For this review, take the finished solid that the model builds, in its own axes (mm). Face numbers are marked on the shaded views. Round coordinates to 2 decimals unless told otherwise and drop trailing zeros. Order: outer loops, then holes, each group sorted by start corner. A loop starts at its lowest first (then second) coordinate and runs counter-clockwise, first axis right, second up.
from build123d import *

# Parameters (mm, degrees)
F0_W      = 45
F0_H      = 21
F0_R      = 2.25
F1_DEPTH  = 2
F2_DEPTH  = 37
F3_R      = 2.25
F4_DEPTH  = 2
F5_DEPTH  = 2
F6_R      = 3.4
F10_DEPTH = 25.29364
F11_R     = 3.4
F12_DEPTH = 13.84716
F13_DEPTH = 13.90348


with BuildPart() as f1:
    # F0 (on Top) → F1 (new body)
    with BuildSketch(Plane.XY):
        Rectangle(F0_W, F0_H)
        with Locations((-15, 0)):
            Circle(F0_R, mode=Mode.SUBTRACT)
        with Locations((15, 0)):
            Circle(F0_R, mode=Mode.SUBTRACT)
    extrude(amount=F1_DEPTH)

    # F0 (on Top) → F2 (join)
    with BuildSketch(Plane.XY):
        Polygon((22.5, 19.5), (22.5, 10.5), (22.5, -10.5), (24.5, -10.5), (24.5, 19.5), align=None)
    extrude(amount=F2_DEPTH)

    # F3 (on face) → F4 (cut)
    with BuildSketch(Plane(origin=(22.5, 0, 0), x_dir=(0, -1, 0), z_dir=(-1, 0, 0))):
        with Locations((0, 30.371862)):
            Circle(F3_R)
    extrude(amount=-F4_DEPTH, mode=Mode.SUBTRACT)

    # F3 (on face) → F5 (cut)
    with BuildSketch(Plane(origin=(22.5, 0, 0), x_dir=(0, -1, 0), z_dir=(-1, 0, 0))):
        with Locations((0, 8.653291)):
            Circle(F3_R)
    extrude(amount=-F5_DEPTH, mode=Mode.SUBTRACT)

    # F9: sweep along a path in F8
    with BuildLine(Plane(origin=(-6.98168, 0, 8.320443), x_dir=(0.766044, 0, 0.642788), z_dir=(0.642788, 0, -0.766044))) as f9_path:
        Line((38.485602, -5.201812), (-16.503841, -5.201812))
    # F6 (on face) → F9 (sweep)
    with BuildSketch(Plane(origin=(22.5, 0, 0), x_dir=(0, -1, 0), z_dir=(-1, 0, 0))):
        with Locations((-6.542337, 33.138294)):
            Circle(F6_R)
        with Locations((6.7, 33.05851)):
            Circle(F6_R)
    sweep(path=f9_path.line)

    # F0 (on Top) → F10 (cut)
    with BuildSketch(Plane.XY):
        Rectangle(F0_W, F0_H)
        with Locations((-15, 0)):
            Circle(F0_R, mode=Mode.SUBTRACT)
        with Locations((15, 0)):
            Circle(F0_R, mode=Mode.SUBTRACT)
    extrude(amount=-F10_DEPTH, mode=Mode.SUBTRACT)

    # F11 (on face) → F12 (join)
    with BuildSketch(Plane.XY.offset(2)):
        with Locations((1.859553, 6.518121)):
            Circle(F11_R)
    extrude(amount=F12_DEPTH)

    # F11 (on face) → F13 (join)
    with BuildSketch(Plane.XY.offset(2)):
        with Locations((1.859553, -6.728277)):
            Circle(F11_R)
    extrude(amount=F13_DEPTH)


solid = f1.part
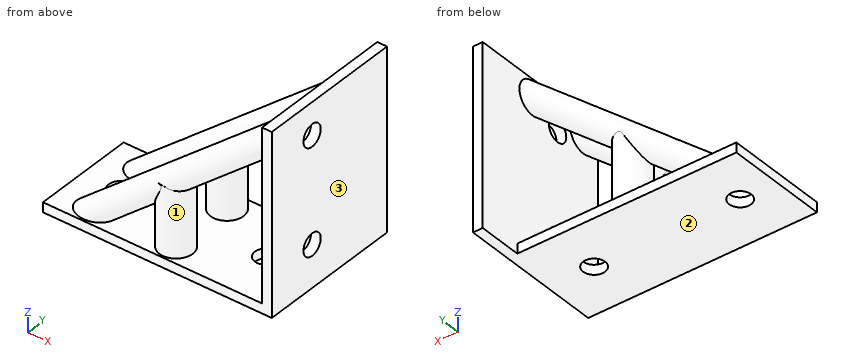
(1) Wall thickness on L1, parallel to Z at x = 23, y = 0; L2, parallel to Y at x = -15, z = 1.3; L3, parallel to X at y = -5.5, z = 8: over which ranges is each line inside the solid? List them lowest first.
(2) Add section B-B on z = 8. Count the separate pieces of the cut face and the enclosed holes in it, plus the area to 3 significant figures.
(3) Add section A-A on y = 0. Give the boundary of the cut face in (x, z), plus the area to 3 significant figures.
(4) Clearance check with flat-ended pins moving along their axes: P1, Ø6.5, axis at x = -4.5, y = 3.5, coming from the +Z side; P2, Ø8, axis at y = 7, z = 12, coming from the -X side; P3, Ø2, axis at x = -8.5, y = 9.5, coming from the +Z side. State where each tip first meets the part, or that it passes through.
(5) Draft analysis for pull direction X (two halves, no side actions). For the marked faces 1, 2 and 3, state which applies: pulls with the +X half, pulls with the -X half, needs draft (parallel to the pull), parting line crosses it, or undercut.
Here are the results:
1. L1: z = 0 to 6.4, 10.9 to 28.12, 32.62 to 37
1. L2: y = -10.5 to -2.25, 2.25 to 10.5
1. L3: x = -11.15 to -3.57, -1.31 to 5.03, 22.5 to 24.5
2. separate pieces: 6
2. enclosed holes: 0
2. area: 211 mm2
3. outline: (-22.5, 0) - (-17.25, 0) - (-17.25, 2) - (-22.5, 2) - close; (-12.75, 0) - (12.75, 0) - (12.75, 2) - (-12.75, 2) - close; (17.25, 0) - (24.5, 0) - (24.5, 6.4) - (22.5, 6.4) - (22.5, 2) - (17.25, 2) - close; (22.5, 10.9) - (24.5, 10.9) - (24.5, 28.12) - (22.5, 28.12) - close; (22.5, 32.62) - (24.5, 32.62) - (24.5, 37) - (22.5, 37) - close
3. area: 128 mm2
4. P1: stops at z = 15.94
4. P2: stops at x = -11.49
4. P3: stops at z = 10.27
5. face 1: undercut
5. face 2: needs draft
5. face 3: pulls with the +X half
